from build123d import *

# Parameters (mm, degrees)
F0_W     = 50.8
F0_H     = 85.725
F1_DEPTH = 3.175
F2_W     = 1.5875
F2_H     = 42.8625
F2_W_2   = 1.6002
F3_DEPTH = 3.176


with BuildPart() as f1:
    # F0 (on Front) → F1 (new body)
    with BuildSketch(Plane.XZ):
        with Locations((-3.192704, 1.555809)):
            Rectangle(F0_W, F0_H)
    extrude(amount=F1_DEPTH)

    # F2 (on face) → F3 (cut, through all)
    with BuildSketch(Plane.XZ.offset(3.175)):
        with Locations((-3.986454, -19.875441)):
            Rectangle(F2_W, F2_H)
        with Locations((-2.392604, -19.875441)):
            Rectangle(F2_W_2, F2_H)
    extrude(amount=-F3_DEPTH, mode=Mode.SUBTRACT)


solid = f1.part
Verification items for the finished model (mm, model axes). A direction names the side the tool comes from. Give positions to 0.01 mm unless a question says otherwise; leave off trailing zeros. Write each loop counter-clockwise with the first axis right and the second up, starting at its lowest first coordinate (ties: lowest second). Pieces come first, ordered by that corner, then holes. Notation, with made-up numbers: M 83,-11 L 134,-11 A22 ccw 134,10 Z; hole C 3.5,60.5 d2. An arc over 180 degrees is marked long. Put each result on its own line as item: value. Start each with the question number.
1. Section check B-B (y = -0.6). Record the cut outline in (x, z).
2. Scan lines: line 1 along X through (y, z) = (-0.25, -13); line 2 along Z through (x, y) = (-4, -0.2). Record each from-to range of solid material in increasing order. Write a range as [from, to].
3. Section check A-A (z = -13.5). Record the cut outline in (x, y) (1 decimal), and give its area (3 significant figures).
4. Go/stop test with a flat-tipped pin: pin 1 Ø1.6 at (x, y) = (-2.5, -2) entering from -Z. Record where the tip stops, or that it passes through.
5. Set-up check for faces 1 (the face through (10, -2, -41.307)), 2 (the face through (-3, -2, 1.556)): record each of +Z, -Z, +X, -X, +Y, -Y from which the full face is reachable in a straight line by a thin tool's end or side.
Answer list:
1. outline: M -28.59,-41.31 L -4.78,-41.31 L -4.78,1.56 L -1.59,1.56 L -1.59,-41.31 L 22.21,-41.31 L 22.21,44.42 L -28.59,44.42 Z
2. line 1: [-28.59, -4.78], [-1.59, 22.21]
2. line 2: [1.56, 44.42]
3. outline: M -28.6,-3.2 L -4.8,-3.2 L -4.8,0 L -28.6,0 Z; M -1.6,-3.2 L 22.2,-3.2 L 22.2,0 L -1.6,0 Z
3. area: 151 mm2
4. pin 1: z = 1.56
5. face 1: -Z, +X, -X, +Y, -Y
5. face 2: -Z, +Y, -Y
